```python
from build123d import *

# Parameters (mm, degrees)
SKETCH_1_W          = 147
SKETCH_1_H          = 147
EXTRUDE_1_DEPTH     = 4
EXTRUDE_2_DEPTH     = 9
SKETCH_3_W          = 103
SKETCH_3_H          = 103
CUT_EXTRUDE_1_DEPTH = 1


with BuildPart() as part:
    # 草图1 → 凸台-拉伸1 (new body)
    with BuildSketch(Plane(origin=(0, 0, 0), x_dir=(1, 0, 0), z_dir=(0, 1, 0))):
        Rectangle(SKETCH_1_W, SKETCH_1_H)
    extrude(amount=EXTRUDE_1_DEPTH)

    # 草图2 → 凸台-拉伸2 (add)
    with BuildSketch(Plane(origin=(0, 4, 0), x_dir=(1, 0, 0), z_dir=(0, 1, 0))):
        with BuildLine():
            Line((49, -64), (-49, -64))
            ThreePointArc((-49, -64), (-59.606601718, -59.606601718), (-64, -49))
            Line((-64, -49), (-64, 49))
            ThreePointArc((-64, 49), (-59.606601718, 59.606601718), (-49, 64))
            Line((-49, 64), (49, 64))
            ThreePointArc((49, 64), (59.606601718, 59.606601718), (64, 49))
            Line((64, 49), (64, -49))
            ThreePointArc((64, -49), (59.606601718, -59.606601718), (49, -64))
        make_face()
    extrude(amount=EXTRUDE_2_DEPTH)

    # 草图3 → 切除-拉伸1 (cut)
    with BuildSketch(Plane.XZ):
        Rectangle(SKETCH_3_W, SKETCH_3_H)
    extrude(amount=-CUT_EXTRUDE_1_DEPTH, mode=Mode.SUBTRACT)


solid = part.part
```
Source: CAD feature listing. Evaluate the final solid. Frame: model axes, mm. A direction names the side the tool comes from. Round coordinates to 2 decimals unless told otherwise and drop trailing zeros. Write each loop counter-clockwise with the first axis right and the second up, starting at its lowest first coordinate (ties: lowest second). Pieces come first, ordered by that corner, then holes. Notation, with made-up numbers: M -29,-10.75 L 18,-10.75 A23 cw 18,28.25 Z; hole C 40.25,-18 d11. An arc over 180 degrees is marked long. Answer as a JSON object with one key per item and string values. Group by question number.
(1) Section query C-C on y = 10.5. Output: boundary loops of the cut face in (x, z).
(2) Reachability of faces 1 (the flat face through (1, 8, 64)), 2 (the flat face through (-1, 8, -64)), 3 (the cylindrical face through (59.72, 8.44, 59.49)), 4 (the cylindrical face through (-59.49, 8.44, 59.72)) from +Z, -Z, +X, -X, +Y, -Y: full face, straight path, thin tool, end or side. Return the list, or none.
(3) Section query A-A on z = -61. Output: boundary loops of the cut face in (x, y).
(4) Ray query, line 1 (Y direction, x = 67, z = 1); line 2 (X direction, y = 5.25, z = -38); line 3 (Y direction, x = -24.5, z = -25). Return the intervals inside material, ascending. Write a range as [from, to].
(5) Section query D-D on z = -17.5. Output: boundary loops of the cut face in (x, y).
(6) Section query B-B on x = 9. Output: boundary loops of the cut face in (y, z), then the cut area to 3 significant figures.
(7) First-contact query: pin 1 (2.5 mm diameter, centred on x = 23, y = 8.5, fed in from -Z); pin 2 (4.5 mm diameter, centred on x = -7.5, y = 9, fed in from +Z); pin 3 (1 mm diameter, centred on x = -52.5, y = 11.5, fed in from -Z). Flat tips, straight axial feed; report the tip coordinate or a pass-through.
(8) Mould query, pull axis X, two halves, no side actions, for faces 5 (the flat face through (-66, 0, -1)), 6 (the flat face through (-1, 1, 1)), 7 (the cylindrical face through (-59.72, 8.44, -59.49)). Classes: +X half, -X half, draft (parallel to the pull), parting line (faces both ways), or undercut.
Computed values:
{
 "1": {"outline": "M -64,-49 A15 ccw -49,-64 L 49,-64 A15 ccw 64,-49 L 64,49 A15 ccw 49,64 L -49,64 A15 ccw -64,49 Z"},
 "2": {"face 1": "+Z, +X, -X, +Y", "face 2": "-Z, +X, -X, +Y", "face 3": "+Z, +X, +Y", "face 4": "+Z, -X, +Y"},
 "3": {"outline": "M -73.5,0 L 73.5,0 L 73.5,4 L 58,4 L 58,13 L -58,13 L -58,4 L -73.5,4 Z"},
 "4": {"line 1": "[0, 4]", "line 2": "[-64, 64]", "line 3": "[1, 13]"},
 "5": {"outline": "M -73.5,0 L -51.5,0 L -51.5,1 L 51.5,1 L 51.5,0 L 73.5,0 L 73.5,4 L 64,4 L 64,13 L -64,13 L -64,4 L -73.5,4 Z"},
 "6": {"outline": "M 0,-73.5 L 4,-73.5 L 4,-64 L 13,-64 L 13,64 L 4,64 L 4,73.5 L 0,73.5 L 0,51.5 L 1,51.5 L 1,-51.5 L 0,-51.5 Z", "area": "1,640 mm^2"},
 "7": {"pin 1": "z = -64", "pin 2": "z = 64", "pin 3": "z = -63.7"},
 "8": {"face 5": "draft", "face 6": "undercut", "face 7": "-X half"}
}
